from build123d import *

# Parameters (mm, degrees)
F0_W            = 6.2
F0_H            = 6.2
F1_DEPTH        = 4.85
F3_DEPTH        = 1.53
F3_COPIES_COUNT = 4
F5_R            = 1.5
F6_DEPTH        = 0.92
F7_SIZE         = 0.2
F8_W            = 0.5751895329
F8_H            = 3.9063365496
F9_DEPTH        = 0.15


# Not quite as in the source:
# - a pattern or mirror of a feature is missing from the dataset's text; its kind, count and spacing are read off the source's solid


with BuildPart() as f1:
    # F0 (on Top) → F1 (new body)
    with BuildSketch(Plane.XY):
        Rectangle(F0_W, F0_H)
    extrude(amount=F1_DEPTH)

    # F2 (on face) → F3 (join)
    with BuildSketch(Plane.XY.offset(4.85)):
        with BuildLine():
            Line((1.1802440276, 2.9), (0, 2.9))
            Line((0, 2.9), (0, 0))
            Line((0, 0), (2.9, 0))
            Line((2.9, 0), (2.9, 1.2403748352))
            Line((2.9, 1.2403748352), (2.6802440276, 1.2403748352))
            ThreePointArc((2.6802440276, 1.2403748352), (1.6195838559, 1.6797146634), (1.1802440276, 2.7403748352))
            Line((1.1802440276, 2.7403748352), (1.1802440276, 2.9))
        make_face()
    f3 = extrude(amount=F3_DEPTH)

    # F3_copies: F3 ×4 about axis
    f3_copies_axis = Axis((0, 0, 0), (0, 0, 1))
    for i in range(1, F3_COPIES_COUNT):
        add(f3.rotate(f3_copies_axis, i * 360 / F3_COPIES_COUNT))

    # F5 (on face) → F6 (join)
    with BuildSketch(Plane.XY.offset(6.38)):
        Circle(F5_R)
    extrude(amount=F6_DEPTH)

    # F7
    f7_edges = [f1.edges().sort_by_distance(p)[0] for p in [
        (-1.5, 0, 7.3),
    ]]
    chamfer(f7_edges, length=F7_SIZE)

    # F8 (on Front) → F9 (join, symmetric)
    with BuildSketch(Plane.XZ):
        with Locations((2.35, -1.5468317252)):
            Rectangle(F8_W, F8_H)
    f9 = extrude(amount=F9_DEPTH, both=True)

    # F9_copies: F9 across plane
    add(f9.mirror(Plane(origin=(0, 0, 0), x_dir=(0, 0, -1), z_dir=(-1, 0, 0))))


solid = f1.part
The listing builds one solid part. Answer for the finished solid, in the listing's coordinates (mm). A direction names the side the tool comes from. Round coordinates to 2 decimals unless told otherwise and drop trailing zeros. Order: outer loops, then holes, each group sorted by start corner. A loop starts at its lowest first (then second) coordinate and runs counter-clockwise, first axis right, second up. Notation, with made-up numbers: M 23,24 L 36,24 A28 ccw 36,55 Z; hole C -30.75,55.5 d1. An arc over 180 degrees is marked long. Answer in a Markdown table with one row per item. Add a question column.
1) The part is cut by section D-D on x = 1.75. Determine the outline of the cut face in (y, z), plus the area to 3 significant figures.
2) Flat-ended cylindrical pins translate along their axes: pin 1 Ø1.5 at (y, z) = (-2, -0.5) entering from -X; pin 2 Ø3 at (x, y) = (0, 0) entering from -Z; pin 3 Ø0.8 at (y, z) = (0, 5.5) entering from +X; pin 4 Ø0.5 at (x, z) = (-0.5, 5.5) entering from +Y. Find the tip coordinate at first contact, or state that the pin passes through.
3) The part is cut by section B-B on y = 0. Determine the outline of the cut face in (x, z).
4) Consider line 1 along X through (y, z) = (0, -0.5); line 2 along Z through (x, y) = (2.5, 2.5); line 3 along Z through (x, y) = (-0.5, 0). Determine where each line is inside the solid, lowest interval first. Write a range as from..to.
5) Determine the mould class of faces 1 (the face through (-2, 2, 4.85)), 2 (the face through (-1.5, 0.07, 6.73)), 3 (the face through (1.6, 1.7, 5.6)) for opening direction X: pulls with the +X half, pulls with the -X half, needs draft (parallel to the pull), parting line crosses it, or undercut.
6) The part is cut by section A-A on x = 0. Determine the outline of the cut face in (y, z), plus the area to 3 significant figures.
7) The part is cut by section C-C on y = 1.75. Determine the outline of the cut face in (x, z).
8) Which of the six approach directions +Z, -Z, +X, -X, +Y, -Y give full straight-line access (tool end or side, diameter ignored) to faces 4 (the face through (1.7, -1.6, 5.6)), 5 (the face through (-2.9, 0, 6)), 6 (the face through (0, -2.9, 6)), 7 (the face through (0, 2.9, 6)), 8 (the face through (2.9, 0, 6))?
Findings below:
| question | item | result |
|---|---|---|
| 1 | outline | M -3.1,0 L 3.1,0 L 3.1,4.85 L 1.56,4.85 L 1.56,6.38 L -1.55,6.38 L -1.55,4.85 L -3.1,4.85 Z |
| 1 | area | 34.8 mm² |
| 2 | pin 1 | stops at x = -3.1 |
| 2 | pin 2 | stops at z = 0 |
| 2 | pin 3 | stops at x = 2.9 |
| 2 | pin 4 | stops at y = 2.9 |
| 3 | outline | M -3.1,0 L -2.64,0 L -2.64,-3.5 L -2.06,-3.5 L -2.06,0 L 2.06,0 L 2.06,-3.5 L 2.64,-3.5 L 2.64,0 L 3.1,0 L 3.1,4.85 L 2.9,4.85 L 2.9,6.38 L 1.5,6.38 L 1.5,7.1 L 1.3,7.3 L -1.3,7.3 L -1.5,7.1 L -1.5,6.38 L -2.9,6.38 L -2.9,4.85 L -3.1,4.85 Z |
| 4 | line 1 | x = -2.64..-2.06, 2.06..2.64 |
| 4 | line 2 | z = 0..4.85 |
| 4 | line 3 | z = 0..7.3 |
| 5 | face 1 | needs draft |
| 5 | face 2 | parting line crosses it |
| 5 | face 3 | pulls with the +X half |
| 6 | outline | M -3.1,0 L 3.1,0 L 3.1,4.85 L 2.9,4.85 L 2.9,6.38 L 1.5,6.38 L 1.5,7.1 L 1.3,7.3 L -1.3,7.3 L -1.5,7.1 L -1.5,6.38 L -2.9,6.38 L -2.9,4.85 L -3.1,4.85 Z |
| 6 | area | 41.7 mm² |
| 7 | outline | M -3.1,0 L 3.1,0 L 3.1,4.85 L 1.55,4.85 L 1.55,6.38 L -1.56,6.38 L -1.56,4.85 L -3.1,4.85 Z |
| 8 | face 4 | +Z, +X, -Y |
| 8 | face 5 | +Z, -X, +Y, -Y |
| 8 | face 6 | +Z, +X, -X, -Y |
| 8 | face 7 | +Z, +X, -X, +Y |
| 8 | face 8 | +Z, +X, +Y, -Y |
